Geometry check sheet. Reference: drawing and pictorial views, mm from the part's lowest x, y, z. Coordinates: 2 decimals unless noted, no trailing zeros. Write each loop counter-clockwise with the first axis right and the second up, starting at its lowest first coordinate (ties: lowest second). Pieces come first, ordered by that corner, then holes. Notation, with made-up numbers: M 18.5,56 L 54.5,56 A31 cw 54.5,82 Z; hole C 33.5,-15.75 d4. An arc over 180 degrees is marked long. One line per item, written item: value.
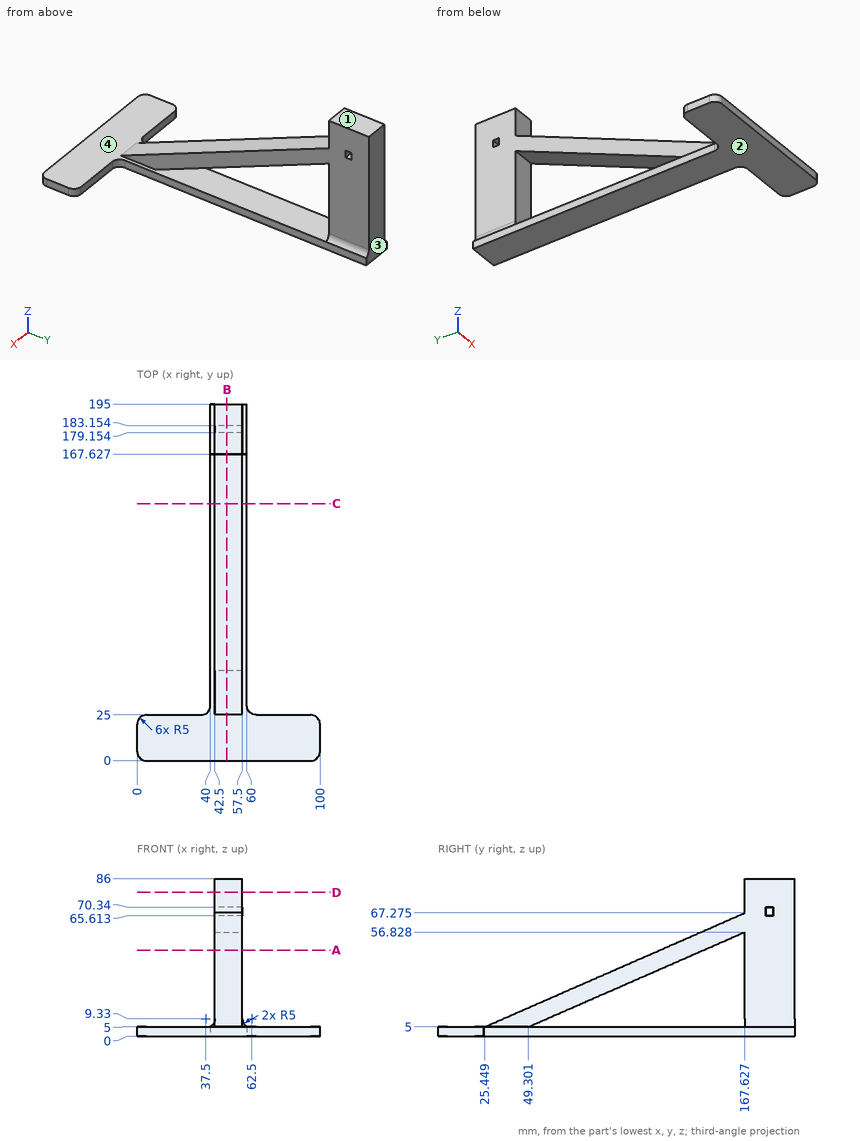
Item 1: Cross-section at B-B, the plane x = 49. Give the number of separate pieces and of enclosed holes in the cut face, and give its area (3 significant figures).
The answers:
separate pieces: 1
enclosed holes: 2
area: 4,530 mm²
Item 2: Draft check along Z on the marked faces 1, 2, 3 and 4. Enter one of: released by +Z, released by -Z, zero draft, split by the parting line, or undercut.
The answers:
face 1: released by +Z
face 2: released by -Z
face 3: zero draft
face 4: undercut
Item 3: Cross-section at C-C, the plane y = 140.5. Enter the section's corners in (x, z).
The answers:
outline: M 40,0 L 60,0 L 60,5 L 40,5 Z; M 42.5,44.95 L 57.5,44.95 L 57.5,55.39 L 42.5,55.39 Z
Item 4: Cross-section at A-A, the plane z = 47. Enter the section's corners in (x, y).
The answers:
outline: M 42.5,121.34 L 57.5,121.34 L 57.5,145.19 L 42.5,145.19 Z; M 42.5,167.63 L 57.5,167.63 L 57.5,195 L 42.5,195 Z
Item 5: Scan lines: line 1 (X direction, y = 168, z = 54.5); line 2 (Y direction, x = 45, z = 29.5) (1 decimal); line 3 (Y direction, x = 43.5, z = 72). Record each from-to range of solid material in increasing order.
The answers:
line 1: x = 42.5 to 57.5
line 2: y = 81.4 to 105.2, 167.6 to 195
line 3: y = 167.63 to 195
Item 6: Go/stop test with flat-tipped pins: P1, Ø1.5, axis at y = 118, z = 2.5, coming from the +X side; P2, Ø6, axis at x = 49.5, z = 38.5, coming from the -Y side (1 decimal); P3, Ø4, axis at y = 33, z = 10, coming from the +X side; P4, Ø1.2, axis at x = 52, y = 182, coming from the -Z side. Record where each tip stops, or that it passes through.
The answers:
P1: stops at x = 60
P2: stops at y = 95.1
P3: stops at x = 57.5
P4: stops at z = 0
Item 7: Cross-section at D-D, the plane z = 78.5. Enter the section's corners in (x, y), and give its area (3 significant figures).
The answers:
outline: M 42.5,167.63 L 57.5,167.63 L 57.5,195 L 42.5,195 Z
area: 411 mm²
